Verification items for the finished model (mm, model axes). Round coordinates to 2 decimals unless told otherwise and drop trailing zeros. Write each loop counter-clockwise with the first axis right and the second up, starting at its lowest first coordinate (ties: lowest second). Pieces come first, ordered by that corner, then holes. Notation, with made-up numbers: (63.25, 47) -> (85.25, 47) arc R23 cw to (85.25, 75) -> close; hole circle Ø2 at (-11, -37.5). An arc over 180 degrees is marked (long way). Use CSV: the item, a comma, the result in double quotes.
```python
from build123d import *

# Parameters (mm, degrees)
SKETCH1_R           = 65.5
SKETCH1_R_2         = 55.5
BOSS_EXTRUDE1_DEPTH = 15
CIRPATTERN1_COUNT   = 8


with BuildPart() as part:
    # Sketch1 → Boss-Extrude1 (new body)
    with BuildSketch(Plane(origin=(0, 0, 0), x_dir=(1, 0, 0), z_dir=(0, 1, 0))):
        Circle(SKETCH1_R)
        Circle(SKETCH1_R_2, mode=Mode.SUBTRACT)
    extrude(amount=-BOSS_EXTRUDE1_DEPTH)

    # Sketch3 → Ø6.0 (6) Diameter Hole2 (revolve, cut)
    with BuildSketch(Plane(origin=(12.141952512, -7.5, 64.364765122), x_dir=(0.98266817, 0, -0.185373321), z_dir=(0, 1, 0))):
        Polygon((0, 0), (0, 67.301581857), (3, 65.499), (3, 0), align=None)
    f_6_0_6_diameter_hole2 = revolve(axis=Axis((13.319073099, -7.5, 70.604708), (-0.185373321, 0, -0.98266817)), mode=Mode.SUBTRACT)

    # CirPattern1: Ø6.0 (6) Diameter Hole2 ×8 about axis
    cirpattern1_axis = Axis((0, 0, 0), (0, 1, 0))
    for i in range(1, CIRPATTERN1_COUNT):
        add(f_6_0_6_diameter_hole2.rotate(cirpattern1_axis, i * 360 / CIRPATTERN1_COUNT), mode=Mode.SUBTRACT)


solid = part.part
```
Q1. Section check B-B (x = 0). Record the cut outline in (y, z), plus the area to 3 significant figures.
Filled in:
outline,"(-15, -65.5) -> (0, -65.5) -> (0, -55.5) -> (-15, -55.5) -> close; (-15, 55.5) -> (0, 55.5) -> (0, 65.5) -> (-15, 65.5) -> close"
area,"300 mm²"
Q2. Mould release check, pull along Y, two halves, no side actions. Record for faces 1 (the flat face through (-54, 0, -15)), 2 (the flat face through (-54, -15, -15)), 3 (the cylindrical face through (-34.66, -4.57, 49.63)): released by +Y, released by -Y, zero draft, split by the parting line, or undercut.
Filled in:
face 1,"released by +Y"
face 2,"released by -Y"
face 3,"undercut"
Q3. Section check C-C (y = -3). Record the cut outline in (x, z), plus the area to 3 significant figures.
Filled in:
outline,"circle Ø131 at (0, 0); hole circle Ø111 at (0, 0)"
area,"3,800 mm²"
Q4. Section check D-D (z = 52). State how many separate pieces and enclosed holes the cut face has, plus the area to 3 significant figures.
Filled in:
separate pieces,"2"
enclosed holes,"1"
area,"579 mm²"
Q5. Go/stop test with flat-tipped pins: P1, Ø1.5, axis at x = -32, y = -3, coming from the -Z side; P2, Ø2, axis at y = -4.5, z = -43, coming from the -X side; P3, Ø3, axis at x = -16, y = -7.5, coming from the +Z side. Record where each tip stops, or that it passes through.
Filled in:
P1,"z = -57.56"
P2,"x = -50.26"
P3,"z = 63.87"
Q6. Material ranges on L1, parallel to X at y = -9, z = 0; L2, parallel to Z at x = 47.5, y = -10, recorded low to high.
Filled in:
L1,"-65.5 to -55.5, 55.5 to 65.5"
L2,"-45.1 to -28.71, 28.71 to 30.42, 34.43 to 45.1"
Q7. Section check A-A (z = 0). Record the cut outline in (x, y), plus the area to 3 significant figures.
Filled in:
outline,"(-65.5, -15) -> (-55.5, -15) -> (-55.5, 0) -> (-65.5, 0) -> close; (55.5, -15) -> (65.5, -15) -> (65.5, 0) -> (55.5, 0) -> close"
area,"300 mm²"
